Verification items for the finished model (mm, model axes). A direction names the side the tool comes from. Give positions to 0.01 mm unless a question says otherwise; leave off trailing zeros. Write each loop counter-clockwise with the first axis right and the second up, starting at its lowest first coordinate (ties: lowest second). Pieces come first, ordered by that corner, then holes. Notation, with made-up numbers: (3.25, 22) -> (9.25, 22) arc R28 cw to (9.25, 49) -> close; hole circle Ø9 at (-24, 27.25). An arc over 180 degrees is marked (long way). Use one line per item in the form item = value. Start each with the question number.
(1) Depth check by flat-ended pin: pin 1 Ø6 at (x, y) = (53.5, 5) entering from -Z; pin 2 Ø2 at (y, z) = (4.5, 4) entering from -X. Enter the tip coordinate at first touch or a pass-through.
(2) Section check A-A, the plane x = 262. Record the cut outline in (y, z) (3 decimals), plus the area to 3 significant figures.
(3) Set-up check for faces 1 (the face through (-6.12, -0.69, -3.1)), 2 (the face through (315.925, 0, 0)): record each of +Z, -Z, +X, -X, +Y, -Y from which the full face is reachable in a straight line by a thin tool's end or side.
(4) Scan lines: L1, parallel to X at y = 1, z = -8.5; L2, parallel to X at y = 2.5, z = 1; L3, parallel to Z at x = 209.5, y = 1.25. Record each from-to range of solid material in increasing order.
Autodesk Inventor part; units mm, degrees
ref_plane "dia1_XY" through (0, 3.175, 0) normal (1, 0, 0) x (0, 0, -1)
ref_plane "dia1_YZ" through (0, 3.175, 0) normal (0, 0, -1) x (0, 1, 0)
ref_plane "dia1_ZX" through (0, 3.175, 0) normal (0, 1, 0) x (1, 0, 0)
sketch "Sketch_1" plane through (0, 0, 0) normal (0, 0, 1) x (1, 0, 0)
  line L0 (315.9252, 0) -> (0, 0)
  line L1 (0, 0) -> (0, 3.175)
  line L2 (0, 3.175) -> (294.4876, 3.175)
  line L3 (294.4876, 3.175) -> (294.4876, 9.6203)
  line L4 (294.4876, 9.6203) -> (315.9252, 9.6203)
  line L5 (315.9252, 9.6203) -> (315.9252, 0)
  line L6 (315.9252, 0) -> (0, 0)
revolve "Revolution1" add sketch "Sketch_1" angle 360 about axis through (315.9252, 0, 0) along (1, 0, 0)
sketch "Sketch_3" plane through (0, 0, 0) normal (0, 0, 1) x (1, 0, 0)
  line L0 (0, 0) -> (-12.7, 0)
  line L1 (-12.7, 0) -> (-12.7, 2.634)
  line L2 (-12.7, 2.634) -> (-12.159, 3.175)
  line L3 (-12.159, 3.175) -> (0, 3.175)
  line L4 (0, 3.175) -> (0, 0)
  line L5 (0, 0) -> (-12.7, 0)
revolve "Revolution2" add sketch "Sketch_3" angle 360 about axis through (0, 0, 0) along (1, 0, 0)
thread "Thread1"
sketch "Sketch_30" plane through (0, 0, 0) normal (0, 0, 1) x (1, 0, 0)
  line L0 (0, 0) -> (-0.254, 0)
  line L1 (-0.254, 2.921) -> (0, 2.921)
  line L2 (0, 2.921) -> (0, 3.429)
  line L3 (0, 3.429) -> (-0.254, 3.429)
  line L4 (-0.254, 3.429) -> (-0.254, 2.921)
revolve "Revolution3" cut sketch "Sketch_30" angle 360 about axis through (0, 0, 0) along (1, 0, 0)
ref_plane "dia1_XY" through (0, 3.175, 0) normal (1, 0, 0) x (0, 0, -1)
ref_plane "dia1_YZ" through (0, 3.175, 0) normal (0, 0, -1) x (0, 1, 0)
ref_plane "dia1_ZX" through (0, 3.175, 0) normal (0, 1, 0) x (1, 0, 0)
ref_plane "dia12_XY" through (0, 0, 10.9537) normal (1, 0, 0) x (0, 0, -1)
ref_plane "dia12_YZ" through (0, 0, 10.9537) normal (0, 0, -1) x (0, 1, 0)
ref_plane "dia12_ZX" through (0, 0, 10.9537) normal (0, 1, 0) x (1, 0, 0)
ref_plane "dia2_XY" through (0, -3.175, 0) normal (1, 0, 0) x (0, 0, -1)
ref_plane "dia2_YZ" through (0, -3.175, 0) normal (0, 0, -1) x (0, 1, 0)
ref_plane "dia2_ZX" through (0, -3.175, 0) normal (0, 1, 0) x (1, 0, 0)
ref_plane "dia22_XY" through (0, 0, -10.9537) normal (1, 0, 0) x (0, 0, -1)
ref_plane "dia22_YZ" through (0, 0, -10.9537) normal (0, 0, -1) x (0, 1, 0)
ref_plane "dia22_ZX" through (0, 0, -10.9537) normal (0, 1, 0) x (1, 0, 0)
ref_plane "rl1_XY" through (-12.7, 0, 0) normal (1, 0, 0) x (0, 0, -1)
ref_plane "rl1_YZ" through (-12.7, 0, 0) normal (0, 0, -1) x (0, 1, 0)
ref_plane "rl1_ZX" through (-12.7, 0, 0) normal (0, 1, 0) x (1, 0, 0)
ref_plane "rl2_XY" through (0, 0, 0) normal (1, 0, 0) x (0, 0, -1)
ref_plane "rl2_YZ" through (0, 0, 0) normal (0, 0, -1) x (0, 1, 0)
ref_plane "rl2_ZX" through (0, 0, 0) normal (0, 1, 0) x (1, 0, 0)
ref_plane "rod_cp_XY" through (0, 0, 0) normal (1, 0, 0) x (0, 0, -1)
ref_plane "rod_cp_YZ" through (0, 0, 0) normal (0, 0, -1) x (0, 1, 0)
ref_plane "rod_cp_ZX" through (0, 0, 0) normal (0, 1, 0) x (1, 0, 0)
ref_plane "thd1_XY" through (-12.7, 3.175, 0) normal (1, 0, 0) x (0, 0, -1)
ref_plane "thd1_YZ" through (-12.7, 3.175, 0) normal (0, 0, -1) x (0, 1, 0)
ref_plane "thd1_ZX" through (-12.7, 3.175, 0) normal (0, 1, 0) x (1, 0, 0)
ref_plane "thd2_XY" through (-12.7, -3.175, 0) normal (1, 0, 0) x (0, 0, -1)
ref_plane "thd2_YZ" through (-12.7, -3.175, 0) normal (0, 0, -1) x (0, 1, 0)
ref_plane "thd2_ZX" through (-12.7, -3.175, 0) normal (0, 1, 0) x (1, 0, 0)
ref_plane "to_rod_clevis_XY" through (-16.764, 0, 0) normal (1, 0, 0) x (0, 0, -1)
ref_plane "to_rod_clevis_YZ" through (-16.764, 0, 0) normal (0, 0, -1) x (0, 1, 0)
ref_plane "to_rod_clevis_ZX" through (-16.764, 0, 0) normal (0, 1, 0) x (1, 0, 0)
properties part number "C-0410-DP0_rod"
Completed:
q1.pin_1 = -2.47
q1.pin_2 = 294.49
q2.outline = circle Ø6.35 at (0, 0)
q2.area = 31.7 mm²
q3.face_1 = -X
q3.face_2 = +Z, -Z, +X, +Y, -Y
q4.L1 = 294.49 to 315.93
q4.L2 = -12.64 to 315.93
q4.L3 = -2.92 to 2.92
